For this review, take the finished solid that the model builds, in its own axes (mm). A direction names the side the tool comes from. Give positions to 0.01 mm unless a question says otherwise; leave off trailing zeros. Loops run counter-clockwise (first coordinate to the right, second up) from the corner with the lowest first, then second, coordinate; pieces in that order, holes last. Notation, with made-up numbers: (-31.75, 66) - (5.25, 66) arc R31 cw to (5.25, 104) - close; hole circle Ø10 at (2.25, -17.75). An arc over 180 degrees is marked (long way). Answer in a Markdown table with one row per item.
```python
from build123d import *

# Parameters (mm, degrees)
F1_DEPTH       = 25
F3_D           = 3.7
F3_CBORE_D     = 6.9
F3_CBORE_DEPTH = 4
F5_DEPTH       = 4
F7_DEPTH       = 4
F9_D           = 4.2
F9_DEPTH       = 4
F11_D          = 3.4
F11_DEPTH      = 4
F12_SIZE       = 0.2


with BuildPart() as f1:
    # F0 (on Top) → F1 (new body)
    with BuildSketch(Plane.XY):
        Polygon((7.5, -7.5), (7.5, 0), (7.5, 7.5), (-7.5, 7.5), (-7.5, -7.5), align=None)
    extrude(amount=F1_DEPTH)

    # F3 (through all)
    with Locations(Plane.XY.offset(25)):
        with Locations((0, 0)):
            CounterBoreHole(F3_D / 2, F3_CBORE_D / 2, F3_CBORE_DEPTH)

    # F4 (on face) → F5 (join)
    with BuildSketch(Plane(origin=(0, 7.5, 0), x_dir=(-1, 0, 0), z_dir=(0, 1, 0))):
        with BuildLine():
            Line((-7.5, 25), (7.5, 25))
            Line((7.5, 25), (7.5, 35))
            ThreePointArc((7.5, 35), (6, 30.5), (2.1, 27.8))
            Line((2.1, 27.8), (-7.5, 25))
        make_face()
        with BuildLine():
            ThreePointArc((2.1, 27.8), (6, 30.5), (7.5, 35))
            ThreePointArc((7.5, 35), (-6, 39.5), (2.1, 27.8))
        make_face()
    extrude(amount=-F5_DEPTH)

    # F6 (on face) → F7 (join)
    with BuildSketch(Plane.XZ.offset(7.5)):
        with BuildLine():
            ThreePointArc((7.5, 35), (0, 42.5), (-7.5, 35))
            ThreePointArc((-7.5, 35), (-6, 30.5), (-2.1, 27.8))
            ThreePointArc((-2.1, 27.8), (4.5, 29), (7.5, 35))
        make_face()
        with BuildLine():
            Line((-7.5, 35), (-7.5, 25))
            Line((-7.5, 25), (7.5, 25))
            Line((7.5, 25), (-2.1, 27.8))
            ThreePointArc((-2.1, 27.8), (-6, 30.5), (-7.5, 35))
        make_face()
    extrude(amount=-F7_DEPTH)

    # F9
    with Locations(Plane.XZ.offset(7.5)):
        with Locations((0, 35)):
            Hole(F9_D / 2, depth=F9_DEPTH)

    # F11
    with Locations(Plane(origin=(0, 7.5, 0), x_dir=(-1, 0, 0), z_dir=(0, 1, 0))):
        with Locations((0, 35)):
            Hole(F11_D / 2, depth=F11_DEPTH)

    # F12
    f12_edges = [f1.edges().sort_by_distance(p)[0] for p in [
        (7.5, -7.5, 12.5),
        (7.5, 7.5, 12.5),
    ]]
    chamfer(f12_edges, length=F12_SIZE)


solid = f1.part
```
1. Mouldability with a two-part tool opening along X and no side actions: class faces 1 (the face through (-0.37, 5.47, 33.34)), 2 (the face through (-7.5, 0, 14)), 3 (the face through (0, 7.5, 22)) as released by +X, released by -X, zero draft, split by the parting line, or undercut.
Values:
| item | result |
|---|---|
| face 1 | undercut |
| face 2 | released by -X |
| face 3 | zero draft |
2. We need section D-D, the plane x = 0. Count the separate pieces of the cut face and the enclosed holes in it, and give its area (3 significant figures).
Values:
| item | result |
|---|---|
| separate pieces | 6 |
| enclosed holes | 0 |
| area | 377 mm^2 |
3. Clearance check with flat-ended pins moving along their axes: pin 1 (2 mm diameter, centred on x = 1.5, y = 1.5, fed in from +Z); pin 2 (3.5 mm diameter, centred on x = 1.5, y = -1, fed in from +Z); pin 3 (2 mm diameter, centred on x = 0, y = 0, fed in from -Z). State where each tip first meets the part, or that it passes through.
Values:
| item | result |
|---|---|
| pin 1 | stops at z = 21 |
| pin 2 | stops at z = 25 |
| pin 3 | passes through |
4. We need section A-A, the plane y = 0. Give the boundary of the cut face in (x, z), and give its area (3 significant figures).
Values:
| item | result |
|---|---|
| outline | (-7.5, 0) - (-1.85, 0) - (-1.85, 21) - (-3.45, 21) - (-3.45, 25) - (-7.5, 25) - close; (1.85, 0) - (7.5, 0) - (7.5, 25) - (3.45, 25) - (3.45, 21) - (1.85, 21) - close |
| area | 270 mm^2 |
5. We need section B-B, the plane z = 8. Give the boundary of the cut face in (x, y), and give its area (3 significant figures).
Values:
| item | result |
|---|---|
| outline | (-7.5, -7.5) - (7.3, -7.5) - (7.5, -7.3) - (7.5, 7.3) - (7.3, 7.5) - (-7.5, 7.5) - close; hole circle Ø3.7 at (0, 0) |
| area | 214 mm^2 |
6. We need section C-C, the plane z = 37.5. Give the boundary of the cut face in (x, y).
Values:
| item | result |
|---|---|
| outline | (-7.07, -7.5) - (7.07, -7.5) - (7.07, -3.5) - (-7.07, -3.5) - close; (-7.07, 3.5) - (7.07, 3.5) - (7.07, 7.5) - (-7.07, 7.5) - close |
7. Wall thickness on line 1 (Y direction, x = -5.5, z = 26); line 2 (Y direction, x = 0, z = 6.75); line 3 (X direction, y = -1.25, z = 7): over which ranges is each line inside the solid? List them lowest first. Write a range as [from, to].
Values:
| item | result |
|---|---|
| line 1 | y = [-7.5, -3.5], [3.5, 7.5] |
| line 2 | y = [-7.5, -1.85], [1.85, 7.5] |
| line 3 | x = [-7.5, -1.36], [1.36, 7.5] |
8. For faces 4 (the face through (-2, 3, 25)), 5 (the face through (-0.45, 3.42, 23.03)), 6 (the face through (0.46, -5.47, 32.95)), 7 (the face through (7.5, 0, 12)), list the 3-axis set-ups (+Z, -Z, +X, -X, +Y, -Y) from which the entire face can be reached by the end or side of a thin tool; tool diameter is ignored.
Values:
| item | result |
|---|---|
| face 4 | +Z, +X, -X |
| face 5 | +Z |
| face 6 | -Y |
| face 7 | +Z, -Z, +X, +Y, -Y |
